Here's how the part is built. I have some questions about the finished solid (model axes, mm). A direction names the side the tool comes from. Round coordinates to 2 decimals unless told otherwise and drop trailing zeros. Order: outer loops, then holes, each group sorted by start corner. A loop starts at its lowest first (then second) coordinate and runs counter-clockwise, first axis right, second up. Notation, with made-up numbers: M 25.25,88.25 L 80.25,88.25 A15 cw 80.25,98.25 Z; hole C 55.25,-6.75 d2. An arc over 180 degrees is marked long. Write item = value, one per line. Start each with the question number.
Item 1: I want a section at A-A, the plane x = 20.5. List the corners of the cut face in (y, z) for me.
Item 2: I want a section at D-D, the plane z = -22. List the corners of the cut face in (x, y) for me.
Item 3: I'm going to push flat-ended pins straight in: P1, Ø8, axis at x = 20.5, y = 58, coming from the +Z side; P2, Ø10.5, axis at x = 17, z = -36, coming from the +Y side; P3, Ø6, axis at x = 22.62, y = 53.69, coming from the +Z side; P4, Ø4, axis at y = 39.22, z = -32.5, coming from the +X side. Where does each tip first touch, or does it pass through?
Item 4: I want a section at C-C, the plane z = -31.5. List the corners of the cut face in (x, y) for me.
Item 5: Please list where these lines run through material, in increasing order: L1, parallel to Z at x = 16.25, y = 57.5; L2, parallel to X at y = 41.25, z = -36.5; L3, parallel to Y at x = 22.25, z = -4.
Item 6: For faces 4 (the face through (19, 42.22, -5)), 5 (the face through (23, 46.22, -21)), 6 (the face through (20.205, 55.9, -24.736)), 7 (the face through (19, 42.22, -38)), which set-ups out of +Z, -Z, +X, -X, +Y, -Y let a thin tool reach every point of the face, with its end or its side?
Item 7: I want a section at B-B, the plane y = 59. List the corners of the cut face in (x, z) for me.
Item 8: We'd pull the mould along X, two halves only. Please class faces 1 (the face through (22, 64.22, -18)), 2 (the face through (20.205, 55.9, -17.736)), 3 (the face through (24.615, 39, -21)): pulls with the +X half, pulls with the -X half, needs draft (parallel to the pull), parting line crosses it, or undercut.
```python
from build123d import *

# Parameters (mm, degrees)
BOSS_EXTRU_1_DEPTH           = 42.5
D_GAGEMENT_M31_D             = 3
BOSS_EXTRU_2_DEPTH           = 18
ESQUISSE7_R                  = 3.27
ENL_V_MAT_EXTRU_1_DEPTH      = 80.23684853
ENL_V_MAT_EXTRU_2_DEPTH      = 87.149089751
ENL_V_MAT_EXTRU_3_DEPTH      = 78.939140419
ENL_V_MAT_EXTRU_3_DEPTH_BACK = 78.939140419
CONG_4_R                     = 8


with BuildPart() as part:
    # Esquisse1 → Boss.-Extru.1 (new body)
    with BuildSketch(Plane(origin=(0, 0, 0), x_dir=(1, 0, 0), z_dir=(0, 0, -1))):
        Polygon((-1.384510159, -46.220398701), (38.615489841, -46.220398701), (38.615489841, -42.220398701), (24.615489841, -42.220398701), (24.615489841, -36.220398701), (12.615489841, -36.220398701), (12.615489841, -42.220398701), (-1.384510159, -42.220398701), align=None)
    extrude(amount=BOSS_EXTRU_1_DEPTH)

    # Dégagement M31 (through all)
    with Locations(Plane(origin=(24.615489841, 0, 0), x_dir=(0, 0, -1), z_dir=(1, 0, 0))):
        with Locations((10, 39.220398701), (32.5, 39.220398701)):
            Hole(D_GAGEMENT_M31_D / 2)

    # Esquisse6 → Boss.-Extru.2 (add)
    with BuildSketch(Plane(origin=(0, 46.220398701, 0), x_dir=(1, 0, 0), z_dir=(0, 1, 0))):
        Polygon((30.615489841, 23.75), (14.615489841, 23.75), (14.615489841, 18.75), (30.615489841, 18.75), (30.615489841, 16.75), (12.615489841, 16.75), (12.615489841, 25.75), (30.615489841, 25.75), align=None)
    extrude(amount=BOSS_EXTRU_2_DEPTH)

    # Esquisse7 → Enlèv. mat.-Extru.1 (cut, through all)
    with BuildSketch(Plane.XY.offset(-16.75)):
        with Locations((22.615489841, 53.690398701)):
            Circle(ESQUISSE7_R)
    extrude(amount=-ENL_V_MAT_EXTRU_1_DEPTH, mode=Mode.SUBTRACT)

    # Esquisse8 → Enlèv. mat.-Extru.2 (cut, through all)
    with BuildSketch(Plane.XY):
        Polygon((30.615489841, 46.220398701), (24.615489841, 42.220398701), (24.615489841, 36.220398701), (12.615489841, 36.220398701), (12.615489841, 42.220398701), (12.615489841, 46.220398701), (-1.384510159, 46.220398701), (-1.384510159, 34.129389344), (38.615489841, 34.129389344), (38.615489841, 46.220398701), align=None)
    extrude(amount=-ENL_V_MAT_EXTRU_2_DEPTH, mode=Mode.SUBTRACT)

    # Esquisse9 → Enlèv. mat.-Extru.3 (cut, two sides: drawn at the far end of the back side and taken through both)
    with BuildSketch(Plane(origin=(24.615489841, 0, 0), x_dir=(0, 0, -1), z_dir=(1, 0, 0)).offset(-ENL_V_MAT_EXTRU_3_DEPTH_BACK)):
        Polygon((16.75, 46.220398701), (12.75, 42.220398701), (0, 42.220398701), (0, 46.220398701), align=None)
        Polygon((25.75, 46.220398701), (29.75, 42.220398701), (42.5, 42.220398701), (42.5, 46.220398701), align=None)
    extrude(amount=ENL_V_MAT_EXTRU_3_DEPTH + ENL_V_MAT_EXTRU_3_DEPTH_BACK, mode=Mode.SUBTRACT)

    # Congé4
    # the kernel refuses this fillet: 8 mm, written as the material it adds along each edge
    with BuildSketch(Plane(origin=(32.899761088, 42.220398701, -12.75), x_dir=(0, 0.7071067811865437, -0.7071067811865512), z_dir=(-1, 0, 0))) as cong_4_piece_1_section:
        with BuildLine():
            CenterArc((CONG_4_R * 0.414213562373, -CONG_4_R), CONG_4_R, 90, 45)
            Line((-CONG_4_R * 0.292893218813, -CONG_4_R * 0.292893218813), (0, 0))
            Line((0, 0), (CONG_4_R * 0.414213562373, 0))
        make_face()
    cong_4_piece_1 = extrude(amount=20.284271247, mode=Mode.PRIVATE)
    cong_4_piece_1 = split(cong_4_piece_1, bisect_by=Plane(origin=(25.761131429, 42.984159759, -13.773553438), z_dir=(-0.5547001962252294, 0.8320502943378435, 0)), keep=Keep.TOP, mode=Mode.PRIVATE)
    cong_4_piece_1 = split(cong_4_piece_1, bisect_by=Plane(origin=(24.615489841, 43.38850385, -13.773553438), z_dir=(1, 0, 0)), keep=Keep.TOP, mode=Mode.PRIVATE)
    add(cong_4_piece_1)
    with BuildSketch(Plane(origin=(24.615489841, 42.220398701, -12.75), x_dir=(0, 0.7071067811865432, -0.7071067811865518), z_dir=(-1, 0, 0))) as cong_4_piece_2_section:
        with BuildLine():
            CenterArc((CONG_4_R * 0.414213562373, -CONG_4_R), CONG_4_R, 90, 45)
            Line((-CONG_4_R * 0.292893218813, -CONG_4_R * 0.292893218813), (0, 0))
            Line((0, 0), (CONG_4_R * 0.414213562373, 0))
        make_face()
    cong_4_piece_2 = extrude(amount=12, mode=Mode.PRIVATE)
    cong_4_piece_2 = split(cong_4_piece_2, bisect_by=Plane(origin=(20.681270928, 39.597586092, -12.548310033), z_dir=(-0.5547001962252294, 0.8320502943378435, 0)), keep=Keep.TOP, mode=Mode.PRIVATE)
    add(cong_4_piece_2)
    with BuildSketch(Plane(origin=(30.615489841, 46.220398701, -16.75), x_dir=(0, 1, 0), z_dir=(-1, 0, 0))) as cong_4_piece_3_section:
        with BuildLine():
            CenterArc((CONG_4_R * 0.414213562373, -CONG_4_R), CONG_4_R, 90, 45)
            Line((-CONG_4_R * 0.292893218813, -CONG_4_R * 0.292893218813), (0, 0))
            Line((0, 0), (CONG_4_R * 0.414213562373, 0))
        make_face()
    cong_4_piece_3 = extrude(amount=18, mode=Mode.PRIVATE)
    cong_4_piece_3 = split(cong_4_piece_3, bisect_by=Plane(origin=(24.307561612, 42.015113215, -16.286257704), z_dir=(-0.5547001962252294, 0.8320502943378435, 0)), keep=Keep.TOP, mode=Mode.PRIVATE)
    add(cong_4_piece_3)
    with BuildSketch(Plane(origin=(12.615489841, 46.220398701, -25.75), x_dir=(0, 1, 0), z_dir=(1, 0, 0))) as cong_4_piece_4_section:
        with BuildLine():
            CenterArc((CONG_4_R * 0.414213562373, -CONG_4_R), CONG_4_R, 90, 45)
            Line((-CONG_4_R * 0.292893218813, -CONG_4_R * 0.292893218813), (0, 0))
            Line((0, 0), (CONG_4_R * 0.414213562373, 0))
        make_face()
    cong_4_piece_4 = extrude(amount=18, mode=Mode.PRIVATE)
    cong_4_piece_4 = split(cong_4_piece_4, bisect_by=Plane(origin=(24.307561612, 42.015113215, -26.213742296), z_dir=(-0.5547001962252294, 0.8320502943378435, 0)), keep=Keep.TOP, mode=Mode.PRIVATE)
    add(cong_4_piece_4)
    with BuildSketch(Plane(origin=(12.615489841, 42.220398701, -29.75), x_dir=(0, 0.7071067811865519, 0.7071067811865432), z_dir=(1, 0, 0))) as cong_4_piece_5_section:
        with BuildLine():
            CenterArc((CONG_4_R * 0.414213562373, -CONG_4_R), CONG_4_R, 90, 45)
            Line((-CONG_4_R * 0.292893218813, -CONG_4_R * 0.292893218813), (0, 0))
            Line((0, 0), (CONG_4_R * 0.414213562373, 0))
        make_face()
    cong_4_piece_5 = extrude(amount=12, mode=Mode.PRIVATE)
    cong_4_piece_5 = split(cong_4_piece_5, bisect_by=Plane(origin=(20.681270928, 39.597586092, -29.951689967), z_dir=(-0.5547001962252294, 0.8320502943378435, 0)), keep=Keep.TOP, mode=Mode.PRIVATE)
    add(cong_4_piece_5)
    with BuildSketch(Plane(origin=(12.615489841, 42.220398701, -29.75), x_dir=(0, 0.7071067811865519, 0.7071067811865432), z_dir=(1, 0, 0))) as cong_4_piece_6_section:
        with BuildLine():
            CenterArc((CONG_4_R * 0.414213562373, -CONG_4_R), CONG_4_R, 90, 45)
            Line((-CONG_4_R * 0.292893218813, -CONG_4_R * 0.292893218813), (0, 0))
            Line((0, 0), (CONG_4_R * 0.414213562373, 0))
        make_face()
    cong_4_piece_6 = extrude(amount=20.284271247, mode=Mode.PRIVATE)
    cong_4_piece_6 = split(cong_4_piece_6, bisect_by=Plane(origin=(25.761131429, 42.984159759, -28.726446562), z_dir=(-0.5547001962252294, 0.8320502943378435, 0)), keep=Keep.TOP, mode=Mode.PRIVATE)
    cong_4_piece_6 = split(cong_4_piece_6, bisect_by=Plane(origin=(24.615489841, 43.38850385, -28.726446562), z_dir=(1, 0, 0)), keep=Keep.TOP, mode=Mode.PRIVATE)
    add(cong_4_piece_6)


solid = part.part
```
Filled in:
q1.outline = M 36.22,-42.5 L 42.22,-42.5 L 42.22,-33.06 A8 cw 44.23,-27.76 A8 cw 49.53,-25.75 L 51.2,-25.75 L 51.2,-23.75 L 46.22,-23.75 L 46.22,-18.75 L 51.2,-18.75 L 51.2,-16.75 L 49.53,-16.75 A8 cw 44.23,-14.74 A8 cw 42.22,-9.44 L 42.22,0 L 36.22,0 Z; M 56.18,-25.75 L 64.22,-25.75 L 64.22,-23.75 L 56.18,-23.75 Z; M 56.18,-18.75 L 64.22,-18.75 L 64.22,-16.75 L 56.18,-16.75 Z; hole C 39.22,-32.5 d3; hole C 39.22,-10 d3
q2.outline = M 12.62,36.22 L 24.62,36.22 L 24.62,42.22 L 30.62,46.22 L 14.62,46.22 L 14.62,64.22 L 12.62,64.22 Z
q3.P1 = -16.75
q3.P2 = 42.56
q3.P3 = through
q3.P4 = 24.62
q4.outline = M 12.62,36.22 L 24.62,36.22 L 24.62,38.1 L 12.62,38.1 Z; M 12.62,40.34 L 24.62,40.34 L 24.62,42.22 L 24.85,42.37 L 12.62,42.37 Z
q5.L1 = -25.75 to -23.75, -18.75 to -16.75
q5.L2 = 12.62 to 24.62
q5.L3 = 36.22 to 42.22
q6.face_4 = +Z, +X, -X, +Y
q6.face_5 = +X, +Y
q6.face_6 = +Z, -Z
q6.face_7 = -Z, +X, -X, +Y
q7.outline = M 12.62,-25.75 L 30.62,-25.75 L 30.62,-23.75 L 14.62,-23.75 L 14.62,-18.75 L 30.62,-18.75 L 30.62,-16.75 L 12.62,-16.75 Z
q8.face_1 = needs draft
q8.face_2 = undercut
q8.face_3 = pulls with the +X half
